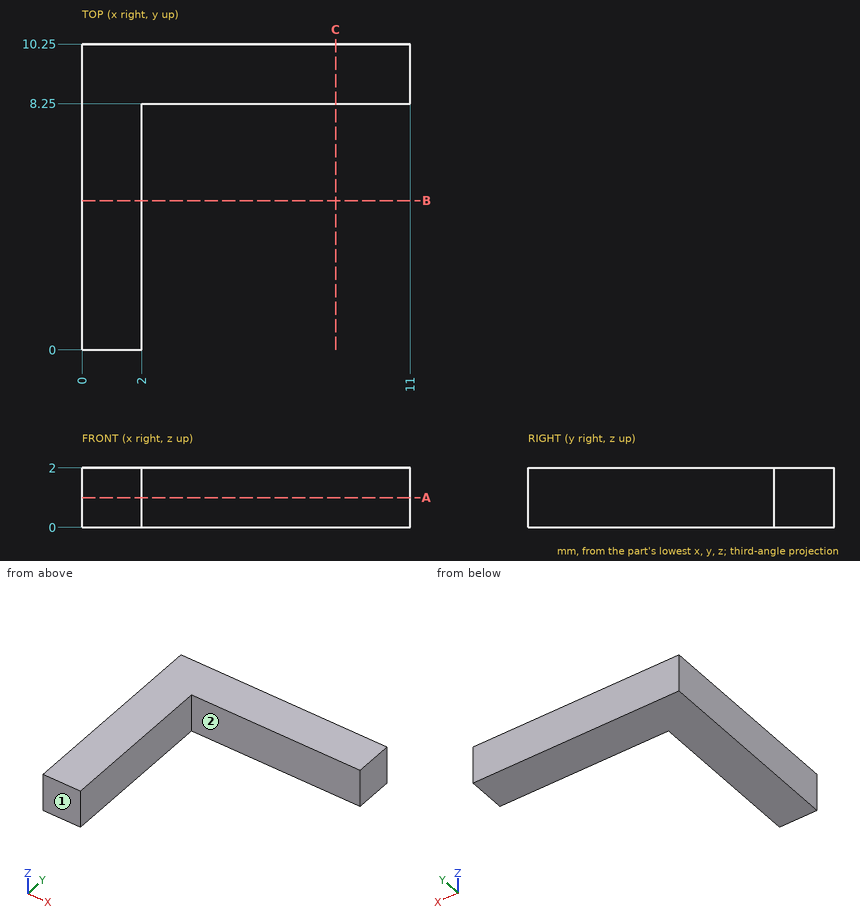
The drawing under review shows one solid part. Ordinate dimensions are in mm from its lowest x, y, z. A direction names the side the tool comes from. Coordinates: 2 decimals unless noted, no trailing zeros. Order: outer loops, then holes, each group sorted by start corner. A loop starts at its lowest first (then second) coordinate and runs counter-clockwise, first axis right, second up. Notation, with made-up numbers: M 81,-9 L 93,-9 A21 cw 93,11 Z; hole C -19,65 d6. An arc over 180 degrees is marked long. Use a Markdown table: item, result.
(1) Add section B-B (y = 5). Give the boundary of the cut face in (x, z).
Worked answers:
| item | result |
|---|---|
| outline | M 0,0 L 2,0 L 2,2 L 0,2 Z |
(2) For P1, Ø3, axis at x = 8.5, y = 5, coming from the -Z side, flat-tipped, find the tip position at first contact; note if it passes through.
Worked answers:
| item | result |
|---|---|
| P1 | passes through |
(3) Add section C-C (x = 8.5). Give the boundary of the cut face in (y, z), then the cut area to 3 significant figures.
Worked answers:
| item | result |
|---|---|
| outline | M 8.25,0 L 10.25,0 L 10.25,2 L 8.25,2 Z |
| area | 4.00 mm2 |
(4) Add section A-A (z = 1). Give the boundary of the cut face in (x, y).
Worked answers:
| item | result |
|---|---|
| outline | M 0,0 L 2,0 L 2,8.25 L 11,8.25 L 11,10.25 L 0,10.25 Z |
(5) Wall thickness on probe 1 along X at (y, z) = (5.5, 1.15); probe 2 along Y at (x, z) = (10.5, 1.65): over which ranges is each line inside the solid? List them lowest first.
Worked answers:
| item | result |
|---|---|
| probe 1 | x = 0 to 2 |
| probe 2 | y = 8.25 to 10.25 |
(6) For the marked faces 1 and 2, list the 3-axis set-ups (+Z, -Z, +X, -X, +Y, -Y) from which the entire face can be reached by the end or side of a thin tool; tool diameter is ignored.
Worked answers:
| item | result |
|---|---|
| face 1 | +Z, -Z, +X, -X, -Y |
| face 2 | +Z, -Z, +X, -Y |
